CAD build for the part. Positions are in the model's coordinates, mm. A direction names the side the tool comes from. Round coordinates to 2 decimals unless told otherwise and drop trailing zeros. Loops run counter-clockwise (first coordinate to the right, second up) from the corner with the lowest first, then second, coordinate; pieces in that order, holes last.
Autodesk Inventor part; units mm, degrees
ref_plane "YZ Plane" through (0, 0, 0) normal (1, 0, 0) x (0, 1, 0)
ref_plane "XZ Plane" through (0, 0, 0) normal (0, 1, 0) x (-1, 0, 0)
ref_plane "XY Plane" through (0, 0, 0) normal (0, 0, 1) x (1, 0, 0)
sketch "Sketch1" plane through (0, 0, 0) normal (0, 0, 1) x (1, 0, 0)
  line L0 (0, 0) -> (-120, 0)
  line L1 (-120, 0) -> (-120, 600)
  line L2 (0, 600) -> (0, 0)
  line L3 (-120, 600) -> (-110, 600)
  line L4 (0, 600) -> (-10, 600)
  line L5 (-60, 582.32) -> (-27.68, 582.32)
  line L6 (-60, 582.32) -> (-92.32, 582.32)
  line L7 (-110, 600) -> (-92.32, 582.32)
  line L8 (-27.68, 582.32) -> (-10, 600)
  line L9 (-120, 600) -> (-110, 600)
  line L10 (-10, 600) -> (0, 600)
  dimension "d0" = 120
  dimension "d1" = 600
  dimension "d3" = 10
  dimension "d4" = 10
  dimension "d5" = 32.32
  dimension "d6" = 32.32
sketch "Sketch2" plane through (0, 0, 0) normal (1, 0, 0) x (0, 1, 0)
  circle A0 centre (0, 0) radius 100
  dimension "d7" = 200
sketch "Sketch3" plane through (0, 0, 0) normal (0, 0, 1) x (1, 0, 0)
  line L0 (0, 0) -> (0, 1416.3001) construction
revolve "Revolution1" add sketch "Sketch1" angle 360 about axis through (0, 0, 0) along (-1, 0, 0)
extrude "Extrusion1" cut sketch "Sketch2" against normal through all
sketch "Sketch4" plane through (0, 0, 0) normal (1, 0, 0) x (0, 0, -1)
  circle A0 centre (0, 0) radius 100
  line L0 (0, 0) -> (25, 0)
  line L1 (25, 96.8246) -> (25, 130)
  line L2 (25, 130) -> (0, 130)
  line L3 (0, 0) -> (-26.4239, 0)
  line L4 (-26.4239, 96.4457) -> (-26.4239, 130)
  line L5 (-26.4239, 130) -> (0, 130)
  dimension "d11" = 25
  dimension "d12" = 130
extrude "Extrusion2" cut sketch "Sketch4" against normal through all contours A0 L4 L5 L2 L1
sketch "Sketch5" plane through (0, 0, 0) normal (1, 0, 0) x (0, 0, -1)
  line L0 (0, 0) -> (350, 0)
  line L1 (0, 0) -> (0, 350)
  line L2 (0, 0) -> (-350, 0)
  line L3 (0, 0) -> (0, -350)
  circle A0 centre (0, 350) radius 37.5
  circle A1 centre (350, 0) radius 37.5
  circle A2 centre (0, -350) radius 37.5
  circle A3 centre (-350, 0) radius 37.5
  dimension "d15" = 350
  dimension "d16" = 350
  dimension "d17" = 350
  dimension "d18" = 350
  dimension "d19" = 75
  dimension "d20" = 75
  dimension "d21" = 75
  dimension "d22" = 75
extrude "Extrusion3" cut sketch "Sketch5" against normal through all
properties part number "P#2_LAB_DINAMICA"
Item 1: Wall check: L1, parallel to Y at x = -85.5, z = 0; L2, parallel to Z at x = -42.5, y = 59; L3, parallel to Z at x = -26, y = 350. Give the ranges that are in metal, low to high.
Verdict:
L1: y = -582.32 to -387.5, -312.5 to -100, 130 to 312.5, 387.5 to 582.32
L2: z = -579.32 to -80.74, 80.74 to 579.32
L3: z = -467.5 to -37.5, 37.5 to 467.5
Item 2: 3-axis set-ups, long thin cutter, end or side, ignore diameter. For faces 1 (the flat face through (-59, 130, 0)), 2 (the flat face through (0, -8, 125)), 3 (the cylindrical face through (-60.45, 555.43, -174.91)): which of +Z, -Z, +X, -X, +Y, -Y reach the whole face in a straight line?
Verdict:
face 1: +X, -X
face 2: +Z, -Z, +X, +Y, -Y
face 3: none
Item 3: Cut at C-C (z = 0). List the corners of the cut face in (x, y).
Verdict:
outline: (-120, -600) - (-110, -600) - (-92.32, -582.32) - (-27.68, -582.32) - (-10, -600) - (0, -600) - (0, -387.5) - (-120, -387.5) - close; (-120, -312.5) - (0, -312.5) - (0, -100) - (-120, -100) - close; (-120, 130) - (0, 130) - (0, 312.5) - (-120, 312.5) - close; (-120, 387.5) - (0, 387.5) - (0, 600) - (-10, 600) - (-27.68, 582.32) - (-92.32, 582.32) - (-110, 600) - (-120, 600) - close
Item 4: Cut at A-A (x = -60). List the corners of the cut face in (y, z), plus the area to 3 significant figures.
Verdict:
outline: circle Ø1164.64 at (0, 0); hole circle Ø75 at (-350, 0); hole circle Ø75 at (0, -350); hole circle Ø75 at (0, 350); hole (96.45, 26.42) arc R100 ccw (long way) to (96.82, -25) - (130, -25) - (130, 26.42) - close; hole circle Ø75 at (350, 0)
area: 1,010,000 mm2
Item 5: Mould opens along Y. For faces 4 (the flat face through (-120, -8, 125)), 5 (the cylindrical face through (-114.93, -78.108, 594.894)), 6 (the cylindrical face through (-59.16, 316.73, -17.3)) say: released by +Y, released by -Y, zero draft, split by the parting line, or undercut.
Verdict:
face 4: zero draft
face 5: split by the parting line
face 6: undercut
Item 6: Cut at B-B (y = 0). List the corners of the cut face in (x, z), plus the area to 3 significant figures.
Verdict:
outline: (-120, -600) - (-110, -600) - (-92.32, -582.32) - (-27.68, -582.32) - (-10, -600) - (0, -600) - (0, -387.5) - (-120, -387.5) - close; (-120, -312.5) - (0, -312.5) - (0, -100) - (-120, -100) - close; (-120, 100) - (0, 100) - (0, 312.5) - (-120, 312.5) - close; (-120, 387.5) - (0, 387.5) - (0, 600) - (-10, 600) - (-27.68, 582.32) - (-92.32, 582.32) - (-110, 600) - (-120, 600) - close
area: 99,100 mm2
Item 7: Flat gauge pins, fed straight in: P1, Ø8, axis at x = -108, y = -78, coming from the +Z side; P2, Ø5, axis at y = 64, z = 402.5, coming from the +X side; P3, Ø4, axis at x = -96, z = 232, coming from the -Y side; P4, Ø8, axis at x = -64, y = 244.5, coming from the -Z side. Where does each tip first touch, or does it go through?
Verdict:
P1: stops at z = 595.35
P2: stops at x = 0
P3: stops at y = -540.46
P4: stops at z = -530.34
